```python
from build123d import *

# Parameters (mm, degrees)
F0_R                 = 60
F1_DEPTH             = 10
F2_SIZE2             = 1.1547005384
F2_SIZE              = 2
F2_2_SIZE2           = 1.1547005384
F2_2_SIZE            = 2
F3_R                 = 4
F4_W                 = 5
F4_H                 = 50
F4_W_2               = 2.6
F4_H_2               = 5.7
F5_DEPTH             = 7.4
F8_D                 = 3.4
F8_DEPTH             = 15
F8_CBORE_D           = 7.5
F8_CBORE_DEPTH       = 3.75
F8_TIP               = 1.0214630523
F8_ON_F7_D           = 3.4
F8_ON_F7_DEPTH       = 15
F8_ON_F7_CBORE_D     = 7.5
F8_ON_F7_CBORE_DEPTH = 3.75
F8_ON_F7_TIP         = 1.0214630523


with BuildPart() as f1:
    # F0 (on Top) → F1 (new body)
    with BuildSketch(Plane.XY):
        with BuildLine():
            Line((-66, 90), (-66, 0))
            ThreePointArc((-66, 0), (0, -66), (66, 0))
            Line((66, 0), (66, 90))
            Line((66, 90), (-66, 90))
        make_face()
        Circle(F0_R, mode=Mode.SUBTRACT)
    extrude(amount=F1_DEPTH)

    # F2
    f2_edges = [f1.edges().sort_by_distance(p)[0] for p in [
        (0, -66, 0),
        (0, -66, 10),
    ]]
    f2_side = f1.faces().sort_by_distance((0, -66, 5))[0]
    chamfer(f2_edges, length=F2_SIZE, length2=F2_SIZE2, reference=f2_side)

    # F2#2
    f2_2_edges = [f1.edges().sort_by_distance(p)[0] for p in [
        (-60, 0, 10),
        (-60, 0, 0),
    ]]
    f2_2_side = f1.faces().sort_by_distance((-60, 0, 5))[0]
    chamfer(f2_2_edges, length=F2_2_SIZE, length2=F2_2_SIZE2, reference=f2_2_side)

    # F3
    f3_edges = [f1.edges().sort_by_distance(p)[0] for p in [
        (0, 90, 10),
    ]]
    fillet(f3_edges, radius=F3_R)

    # F4 (on face) → F5 (cut)
    with BuildSketch(Plane(origin=(0, 0, 0), x_dir=(1, 0, 0), z_dir=(0, 0, -1))):
        with Locations((58.75, -65)):
            Rectangle(F4_W, F4_H)
        with Locations((-58.75, -65)):
            Rectangle(F4_W, F4_H)
        with Locations((-53.95, -80.4)):
            Rectangle(F4_W_2, F4_H_2)
        with Locations((53.95, -80.4)):
            Rectangle(F4_W_2, F4_H_2)
    extrude(amount=-F5_DEPTH, mode=Mode.SUBTRACT)

    # F8
    with Locations(Plane(origin=(-66, 0, 0), x_dir=(0, -1, 0), z_dir=(-1, 0, 0))):
        with Locations((-80.4, 3.5)):
            CounterBoreHole(F8_D / 2, F8_CBORE_D / 2, F8_CBORE_DEPTH, depth=F8_DEPTH)
            with Locations((0, 0, -(F8_DEPTH + F8_TIP / 2))):  # 118° drill point
                Cone(0, F8_D / 2, F8_TIP, mode=Mode.SUBTRACT)

    # F8 on F7
    with Locations(Plane.YZ.offset(66)):
        with Locations((80.4, 3.5)):
            CounterBoreHole(F8_ON_F7_D / 2, F8_ON_F7_CBORE_D / 2, F8_ON_F7_CBORE_DEPTH, depth=F8_ON_F7_DEPTH)
            with Locations((0, 0, -(F8_ON_F7_DEPTH + F8_ON_F7_TIP / 2))):  # 118° drill point
                Cone(0, F8_ON_F7_D / 2, F8_ON_F7_TIP, mode=Mode.SUBTRACT)


solid = f1.part
```
Here's how the part is built. I have some questions about the finished solid (model axes, mm). A direction names the side the tool comes from. Round coordinates to 2 decimals unless told otherwise and drop trailing zeros. Loops run counter-clockwise (first coordinate to the right, second up) from the corner with the lowest first, then second, coordinate; pieces in that order, holes last.
1. For faces 1 (the face through (55.25, 81.1, 5.3)), 2 (the face through (62.25, 82, 4.5)), 3 (the face through (-61.25, 65, 4)), 4 (the face through (-64.151, 80.254, 7.247)), which set-ups out of +Z, -Z, +X, -X, +Y, -Y let a thin tool reach every point of the face, with its end or its side?
Answers:
face 1: -Z
face 2: +X
face 3: -Z, +Y
face 4: -X
2. Thinking about a two-plate mould opening in X: for faces 5 (the face through (1, 90, 3)), 6 (the face through (-59, 40, 4)), 7 (the face through (66, 44, 5)), 8 (the face through (-52.65, 81.1, 5.3)), which applies, released by +X, released by -X, zero draft, split by the parting line, or undercut?
Answers:
face 5: zero draft
face 6: undercut
face 7: released by +X
face 8: undercut
3. If I drill on probe 1 along X at (y, z) = (77, 4.5); probe 2 along Y at (x, z) = (0, 4.55); probe 3 along X at (y, z) = (56, 0.75), over which ranges is the centre line in solid material (lowest first)?
Answers:
probe 1: x = -62.25 to -61.25, -56.25 to 56.25, 61.25 to 62.25
probe 2: y = -66 to -60, 60 to 90
probe 3: x = -65.28 to -61.25, -56.25 to -23.48, 23.48 to 56.25, 61.25 to 65.28
4. Will these pins go through, and if not, where does the flat tip stop? pin 1 (6 mm diameter, centred on y = 80, z = 4, fed in from +X); pin 2 (4 mm diameter, centred on x = 30.5, z = 6, fed in from -Y); pin 3 (5.5 mm diameter, centred on y = 80.4, z = 3.5, fed in from -X).
Answers:
pin 1: stops at x = 62.25
pin 2: stops at y = -59.53
pin 3: stops at x = -62.25
5. Suppose I cut it at A-A, the plane x = 0. Please give me the cut outline in (y, z).
Answers:
outline: (-66, 2) - (-64.85, 0) - (-61.15, 0) - (-60, 2) - (-60, 8) - (-61.15, 10) - (-64.85, 10) - (-66, 8) - close; (60, 2) - (61.15, 0) - (90, 0) - (90, 6) arc R4 ccw to (86, 10) - (61.15, 10) - (60, 8) - close
